Input: part model. Units: mm. Frame: model coordinates. A direction names the side the tool comes from. Coordinates: 2 decimals unless noted, no trailing zeros. Order: outer loops, then holes, each group sorted by start corner. A loop starts at its lowest first (then second) coordinate and runs counter-clockwise, first axis right, second up. Notation, with made-up numbers: M 79,16.5 L 122,16.5 A15 cw 122,32.5 Z; hole C -1.75,-35 d2. An arc over 180 degrees is marked long. One line per item, written item: value.
```python
from build123d import *

# Parameters (mm, degrees)
F0_R        = 15.875
F1_DEPTH    = 50.8
F2_DEPTH    = 31.75
F0_R_2      = 9.525
F3_DEPTH    = 19.05
F4_T1_DEPTH = 61.8868884968


# Not quite as in the source:
# - a fillet or chamfer that OpenCascade refuses, or shapes differently, is made with other operations: its cross-section is extruded or revolved along the edge and cut away or added


with BuildPart() as f1:
    # F0 (on Top) → F1 (new body)
    with BuildSketch(Plane.XY):
        with BuildLine():
            ThreePointArc((-25.9736086209, -23.8194207925), (-16.5833436809, -13.5180364382), (-13.1835957324, 0))
            ThreePointArc((-13.1835957324, 0), (-19.7400794655, 18.2130603251), (-36.4007832324, 28.0682110263))
            ThreePointArc((-36.4007832324, 28.0682110263), (-69.7735217146, -5.6297910447), (-25.9736086209, -23.8194207925))
        make_face()
        with Locations((-41.7585957324, 0)):
            Circle(F0_R, mode=Mode.SUBTRACT)
    extrude(amount=F1_DEPTH)

    # F0 (on Top) → F2 (join)
    with BuildSketch(Plane.XY):
        with BuildLine():
            ThreePointArc((-36.4007832324, 28.0682110263), (-19.7400794655, 18.2130603251), (-13.1835957324, 0))
            ThreePointArc((-13.1835957324, 0), (-16.5833436809, -13.5180364382), (-25.9736086209, -23.8194207925))
            Line((-25.9736086209, -23.8194207925), (11.5255643148, -18.8873356739))
            ThreePointArc((11.5255643148, -18.8873356739), (-10.0006293875, 0.5508668403), (12.6132792676, 18.7121406842))
            Line((12.6132792676, 18.7121406842), (-36.4007832324, 28.0682110263))
        make_face()
    extrude(amount=F2_DEPTH)

    # F0 (on Top) → F3 (join)
    with BuildSketch(Plane.XY):
        with BuildLine():
            ThreePointArc((28.0914042676, 0), (23.7204151122, 12.1420402167), (12.6132792676, 18.7121406842))
            ThreePointArc((12.6132792676, 18.7121406842), (-10.0006293875, 0.5508668403), (11.5255643148, -18.8873356739))
            ThreePointArc((11.5255643148, -18.8873356739), (23.3631665352, -12.5614340563), (28.0914042676, 0))
        make_face()
        with Locations((9.0414042676, 0)):
            Circle(F0_R_2, mode=Mode.SUBTRACT)
    extrude(amount=F3_DEPTH)

    # F4: fillet of radius 5.08 on 2 edges, made by hand

    # F4_s2 → F4_t1 (cut)
    with BuildSketch(Plane.XY.offset(19.05)):
        with BuildLine():
            ThreePointArc((-6.7125365301, 22.4011573214), (-2.7943533432, 18.8544597398), (-4.147891099, 13.7457261624))
            ThreePointArc((-4.147891099, 13.7457261624), (3.6293795146, 18.265061951), (12.6132792676, 18.7121406842))
            Line((12.6132792676, 18.7121406842), (-6.7125365301, 22.4011573214))
        make_face()
        with BuildLine():
            ThreePointArc((-7.9811920904, -21.4529651384), (-3.8645283867, -18.1387075787), (-4.9204686565, -12.9602702306))
            ThreePointArc((-4.9204686565, -12.9602702306), (2.5825344428, -17.921648936), (11.5255643148, -18.8873356739))
            Line((11.5255643148, -18.8873356739), (-7.9811920904, -21.4529651384))
        make_face()
    extrude(amount=F4_T1_DEPTH, mode=Mode.SUBTRACT)


solid = f1.part
```
(1) Cut plane B-B on x = -56.5. Output: boundary loops of the cut face in (y, z).
Data:
outline: M -24.48,0 L -5.89,0 L -5.89,50.8 L -24.48,50.8 Z; M 5.89,0 L 24.48,0 L 24.48,50.8 L 5.89,50.8 Z
(2) Cut plane A-A on z = 5. Output: boundary loops of the cut face in (x, y) (3 decimals), plus the area to 3 significant figures.
Data:
outline: M -36.401,28.068 A28.575 ccw long -25.974,-23.819 L 11.526,-18.887 A19.05 ccw 12.613,18.712 Z; hole C -41.759,0 d31.75; hole C 9.041,0 d19.05
area: 3,190 mm2
(3) Access query for faces 1 (the cylindrical face through (17.84, -3.65, 9.39)), 2 (the cylindrical face through (-10.005, 0.344, 25.311)), 3 (the cylindrical face through (-64.677, -17.066, 25.044)). Directions: +Z, -Z, +X, -X, +Y, -Y. A direction counts if a zero-diameter tool reaches every point of the face in a straight line with its end or side. Return the directions, or none.
Data:
face 1: +Z, -Z
face 2: +Z, +X
face 3: +Z
(4) Cut plane D-D on z = 40.5. Output: boundary loops of the cut face in (x, y) (3 decimals).
Data:
outline: C -41.759,0 d57.15; hole C -41.759,0 d31.75
(5) First-contact query: pin 1 (6 mm diameter, centred on x = -31.5, z = 9.5, fed in from -Y); pin 2 (2 mm diameter, centred on y = 5, z = 24, fed in from -X); pin 3 (11.5 mm diameter, centred on x = 9.04, y = 0, fed in from -Z); pin 4 (4 mm diameter, centred on x = -0.5, y = -1.5, fed in from +Z). Flat tips, straight axial feed; report the tip coordinate or a pass-through.
Data:
pin 1: stops at y = -27.64
pin 2: stops at x = -70.05
pin 3: passes through
pin 4: stops at z = 19.05
(6) Ray query, line 1 (X direction, y = 5.5, z = 15.5); line 2 (Y direction, x = -45.5, z = 12.5); line 3 (Y direction, x = -42, z = 10.5). Return the intervals inside material, ascending. Write a range as from..to.
Data:
line 1: x = -69.8..-56.65, -26.87..1.26, 16.82..27.28
line 2: y = -28.33..-15.43, 15.43..28.33
line 3: y = -28.57..-15.87, 15.87..28.57
(7) Cut plane C-C on y = 11. Output: boundary loops of the cut face in (x, z), plus the area to 3 significant figures.
Data:
outline: M -68.13,0 L -53.2,0 L -53.2,50.8 L -68.13,50.8 Z; M -30.31,0 L 24.59,0 L 24.59,19.05 L -6.51,19.05 L -6.51,31.75 L -15.39,31.75 L -15.39,50.8 L -30.31,50.8 Z
area: 2,390 mm2
(8) Draft query along Y for faces 4 (the flat face through (-11.653, -21.936, 12.125)), 5 (the cylindrical face through (-57.62, 0.7, 25.04)), 6 (the flat face through (-12, 2, 31.75)). Return one class per face: released by +Y, released by -Y, zero draft, split by the parting line, or undercut.
Data:
face 4: released by -Y
face 5: undercut
face 6: zero draft
